Check sheet for the modelled part. Datum: model origin and axes. Units: mm. Give positions to 0.01 mm unless a question says otherwise; leave off trailing zeros. Order: outer loops, then holes, each group sorted by start corner. A loop starts at its lowest first (then second) coordinate and runs counter-clockwise, first axis right, second up.
Item 1: Release check for a two-part mould opening along X. For faces 1 (the cylindrical face through (-0.54, 2.44, -0.14)), 2 (the cylindrical face through (-1.5, 0.07, 1.52)) record: released by +X, released by -X, zero draft, split by the parting line, or undercut.
Item 2: Gauge pin test, flat ends, axial feed: P1, Ø1, axis at x = -2, z = 0, coming from the -Y side; P2, Ø2, axis at x = -1.5, z = 1.5, coming from the +Y side; P3, Ø1, axis at y = 0.5, z = 2.5, coming from the +X side. Record the tip position at first contact, or that the pin passes through.
Item 3: Sectioned sample at C-C on z = 1.35. Record the boundary of the cut face in (x, y), and give its area (3 significant figures).
Item 4: Material ranges on line 1 along Y through (x, z) = (0, 1.9); line 2 along Y through (x, z) = (1.4, -0.5); line 3 along X through (y, z) = (1.2, 0.45), recorded low to high.
Item 5: Sectioned sample at D-D on z = 0.5. Record the boundary of the cut face in (x, y), and give its area (3 significant figures).
Autodesk Inventor part; units mm, degrees
sketch "Skizze1" plane through (0, 0, 0) normal (0, 0, 1) x (1, 0, 0)
  circle A0 centre (0, 0) radius 2.5
  dimension "d0" = 5
extrude "Extrusion1" add sketch "Skizze1" along normal mid plane 2
sketch "Skizze2" plane through (0, 0, 1) normal (0, 0, 1) x (1, 0, 0)
  circle A0 centre (0, 0) radius 2
  dimension "d3" = 4
extrude "Extrusion2" add sketch "Skizze2" along normal blind 2
sketch "Skizze3" plane through (0, 0, 3) normal (0, 0, 1) x (1, 0, 0)
  circle A0 centre (0, 0) radius 1.5
  dimension "d6" = 3
extrude "Extrusion3" cut sketch "Skizze3" against normal blind 5
fillet "Rundung1" radius 1 1 edges at (-1.5, 0, -1)
thread "Gewinde1"
thread "Gewinde2"
fillet "Rundung2" radius 0.25 1 edges at (-2.5, 0, 1)
properties part number "SchleppstangeBefestigungUnten"
Report:
1. face 1: split by the parting line
1. face 2: undercut
2. P1: stops at y = -2
2. P2: stops at y = 2.37
2. P3: stops at x = 2
3. outline: circle Ø4 at (0, 0); hole circle Ø3 at (0, 0)
3. area: 5.50 mm2
4. line 1: y = -2 to -1.5, 1.5 to 2
4. line 2: y = -2.07 to -0.84, 0.84 to 2.07
4. line 3: x = -2.19 to -0.9, 0.9 to 2.19
5. outline: circle Ø5 at (0, 0); hole circle Ø3 at (0, 0)
5. area: 12.6 mm2
